from build123d import *

# Parameters (mm, degrees)
SKETCH2_R     = 0.7
CHAMFER1_SIZE = 0.3


with BuildPart() as part:
    # Sweep1: sweep along a path in Sketch1
    with BuildLine(Plane(origin=(0, 0, 0), x_dir=(1, 0, 0), z_dir=(0, 1, 0))) as sweep1_path:
        Line((0, 0), (0, 16))
        ThreePointArc((0, 16), (0.585786438, 17.414213562), (2, 18))
        Line((2, 18), (3.75, 18))
        ThreePointArc((3.75, 18), (5.164213562, 18.585786438), (5.75, 20))
        Line((5.75, 20), (5.75, 29))
    # Sketch2 → Sweep1 (sweep)
    with BuildSketch(Plane.XY):
        Circle(SKETCH2_R)
    sweep(path=sweep1_path.line)

    # Chamfer1
    chamfer1_edges = [part.edges().sort_by_distance(p)[0] for p in [
        (5.05, 0, -29),
    ]]
    chamfer(chamfer1_edges, length=CHAMFER1_SIZE)


solid = part.part
Verification items for the finished model (mm, model axes). A direction names the side the tool comes from. Coordinates: 2 decimals unless noted, no trailing zeros. Order: outer loops, then holes, each group sorted by start corner. A loop starts at its lowest first (then second) coordinate and runs counter-clockwise, first axis right, second up. Notation, with made-up numbers: (79.25, 78.25) -> (93.25, 78.25) arc R17 cw to (93.25, 89.25) -> close; hole circle Ø3 at (17, 24.25). An arc over 180 degrees is marked (long way). Put each result on its own line as item: value. Start each with the question number.
1. Access from +Z, -Z, +X, -X, +Y, -Y to the whole of each face (thin tool, end or side, straight path). Record for faces 1 (the cylindrical face through (-0.7, 0, -8.1)), 2 (the cylindrical face through (2.887, -0.21, -17.332)), 3 (the cylindrical face through (5.05, -0.03, -24.41)).
2. Cross-section at C-C, the plane z = -26.75. Record the boundary of the cut face in (x, y), then the cut area to 3 significant figures.
3. Material ranges on L1, parallel to Z at x = 4.75, y = -0.6; L2, parallel to Z at x = 1.5, y = 0.3; L3, parallel to Y at x = -0.5, z = -2.75, recorded low to high. Write a range as [from, to].
4. Cross-section at B-B, the plane x = 2.25. Record the boundary of the cut face in (y, z).
5. Cross-section at A-A, the plane y = 0. Record the boundary of the cut face in (x, z).
Computed:
1. face 1: +Z
1. face 2: none
1. face 3: -Z
2. outline: circle Ø1.4 at (5.75, 0)
2. area: 1.54 mm2
3. L1: [-18.7, -17.86]
3. L2: [-18.58, -17.27]
3. L3: [-0.49, 0.49]
4. outline: circle Ø1.4 at (0, -18)
5. outline: (-0.7, -16) arc R2.7 ccw to (2, -18.7) -> (3.75, -18.7) arc R1.3 cw to (5.05, -20) -> (5.05, -28.7) -> (5.35, -29) -> (6.15, -29) -> (6.45, -28.7) -> (6.45, -20) arc R2.7 ccw to (3.75, -17.3) -> (2, -17.3) arc R1.3 cw to (0.7, -16) -> (0.7, 0) -> (-0.7, 0) -> close
